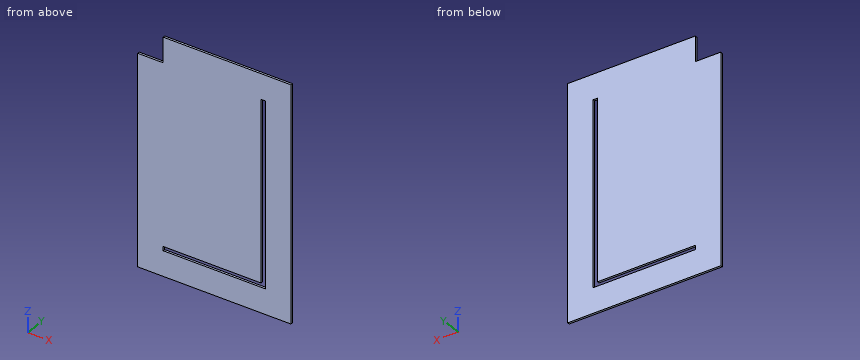
from build123d import *

# Parameters (mm, degrees)
SKETCH2_W           = 228.6
SKETCH2_H           = 355.6
BOSS_EXTRUDE1_DEPTH = 3.175
SKETCH3_W           = 6.35
SKETCH3_H           = 273.05
CUT_EXTRUDE1_DEPTH  = 212.393970172
SKETCH4_W           = 38.1
SKETCH4_H           = 38.1
CUT_EXTRUDE2_DEPTH  = 212.393970172


with BuildPart() as part:
    # Sketch2 → Boss-Extrude1 (new body)
    with BuildSketch(Plane(origin=(0, 0, 0), x_dir=(1, 0, 0), z_dir=(0, 1, 0))):
        Rectangle(SKETCH2_W, SKETCH2_H)
    extrude(amount=BOSS_EXTRUDE1_DEPTH)

    # Sketch3 → Cut-Extrude1 (cut, through all)
    with BuildSketch(Plane(origin=(0, 3.175, 0), x_dir=(1, 0, 0), z_dir=(0, 1, 0))):
        Polygon((76.2, 139.7), (-76.2, 139.7), (-76.2, 133.35), (69.85, 133.35), (76.2, 133.35), align=None)
        with Locations((73.025, -3.175)):
            Rectangle(SKETCH3_W, SKETCH3_H)
    extrude(amount=-CUT_EXTRUDE1_DEPTH, mode=Mode.SUBTRACT)

    # Sketch4 → Cut-Extrude2 (cut, through all)
    with BuildSketch(Plane(origin=(0, 3.175, 0), x_dir=(1, 0, 0), z_dir=(0, 1, 0))):
        with Locations((-95.25, -158.75)):
            Rectangle(SKETCH4_W, SKETCH4_H)
    extrude(amount=-CUT_EXTRUDE2_DEPTH, mode=Mode.SUBTRACT)


solid = part.part
Verification items for the finished model (mm, model axes). Coordinates: 2 decimals unless noted, no trailing zeros. Order: outer loops, then holes, each group sorted by start corner. A loop starts at its lowest first (then second) coordinate and runs counter-clockwise, first axis right, second up. Notation, with made-up numbers: (82, 78) -> (93, 78) arc R21 ccw to (93, 90) -> close; hole circle Ø7 at (51.5, 63.25). An arc over 180 degrees is marked (long way). Use CSV: the item, a comma, the result in double quotes. Start each with the question number.
Q1. Section check B-B, the plane x = -29.5. Record the cut outline in (y, z) (3 decimals), and give its area (3 significant figures).
Q2. Section check A-A, the plane z = 132.5. Record the cut outline in (x, y) (3 decimals), and give its area (3 significant figures).
Q3. Section check D-D, the plane x = -84. Record the cut outline in (y, z) (3 decimals).
Q4. Section check C-C, the plane y = 1.35. Record the cut outline in (x, z), and give its area (3 significant figures).
Q5. Thickness scan on line 1 along X through (y, z) = (1.7, 78.5); line 2 along Z through (x, y) = (27, 1.05); line 3 along X through (y, z) = (1.8, 148). Record the ranges inside material, lowest first.
Returned:
1,outline,"(0, -177.8) -> (3.175, -177.8) -> (3.175, -139.7) -> (0, -139.7) -> close; (0, -133.35) -> (3.175, -133.35) -> (3.175, 177.8) -> (0, 177.8) -> close"
1,area,"1,110 mm^2"
2,outline,"(-114.3, 0) -> (69.85, 0) -> (69.85, 3.175) -> (-114.3, 3.175) -> close; (76.2, 0) -> (114.3, 0) -> (114.3, 3.175) -> (76.2, 3.175) -> close"
2,area,"706 mm^2"
3,outline,"(0, -177.8) -> (3.175, -177.8) -> (3.175, 139.7) -> (0, 139.7) -> close"
4,outline,"(-114.3, -177.8) -> (114.3, -177.8) -> (114.3, 177.8) -> (-76.2, 177.8) -> (-76.2, 139.7) -> (-114.3, 139.7) -> close; hole (-76.2, -139.7) -> (76.2, -139.7) -> (76.2, 139.7) -> (69.85, 139.7) -> (69.85, -133.35) -> (-76.2, -133.35) -> close"
4,area,"77,100 mm^2"
5,line 1,"x = -114.3 to 69.85, 76.2 to 114.3"
5,line 2,"z = -177.8 to -139.7, -133.35 to 177.8"
5,line 3,"x = -76.2 to 114.3"
